Verification items for this drawing (mm, ordinates from the low corner). Round coordinates to 2 decimals unless told otherwise and drop trailing zeros. Order: outer loops, then holes, each group sorted by start corner. A loop starts at its lowest first (then second) coordinate and runs counter-clockwise, first axis right, second up. Notation, with made-up numbers: (-33.5, 84) - (-23.5, 84) arc R31 ccw to (-23.5, 117) - close; hole circle Ø8 at (38, -18.5). An arc over 180 degrees is marked (long way). Use a Markdown table: item, result. Add a question column.
(1) Gauge pin test, flat end, axial feed: P1, Ø10, axis at x = 15, y = 10, coming from the +Z side. Record the tip position at first contact, or that the pin passes through.
(2) Section check B-B on z = 56.5. Record the boundary of the cut face in (x, y).
(3) Section check C-C on y = 40.5. Record the boundary of the cut face in (x, z).
(4) Section check A-A on x = 70.5. Record the boundary of the cut face in (y, z), then the cut area to 3 significant figures.
(5) Mould release check, pull along Z, two halves, no side actions. Record for the marked faces 1, 2, 3 and 4: released by +Z, released by -Z, zero draft, split by the parting line, or undercut.
(6) Section check D-D on x = 82. Record the boundary of the cut face in (y, z) (1 decimal).
(7) Thickness scan on line 1 along Z through (x, y) = (49, 36) (1 decimal); line 2 along X through (y, z) = (35.5, 25); line 3 along X through (y, z) = (27, 61.5) (1 decimal). Record the ranges inside material, lowest first. Write a range as [from, to].
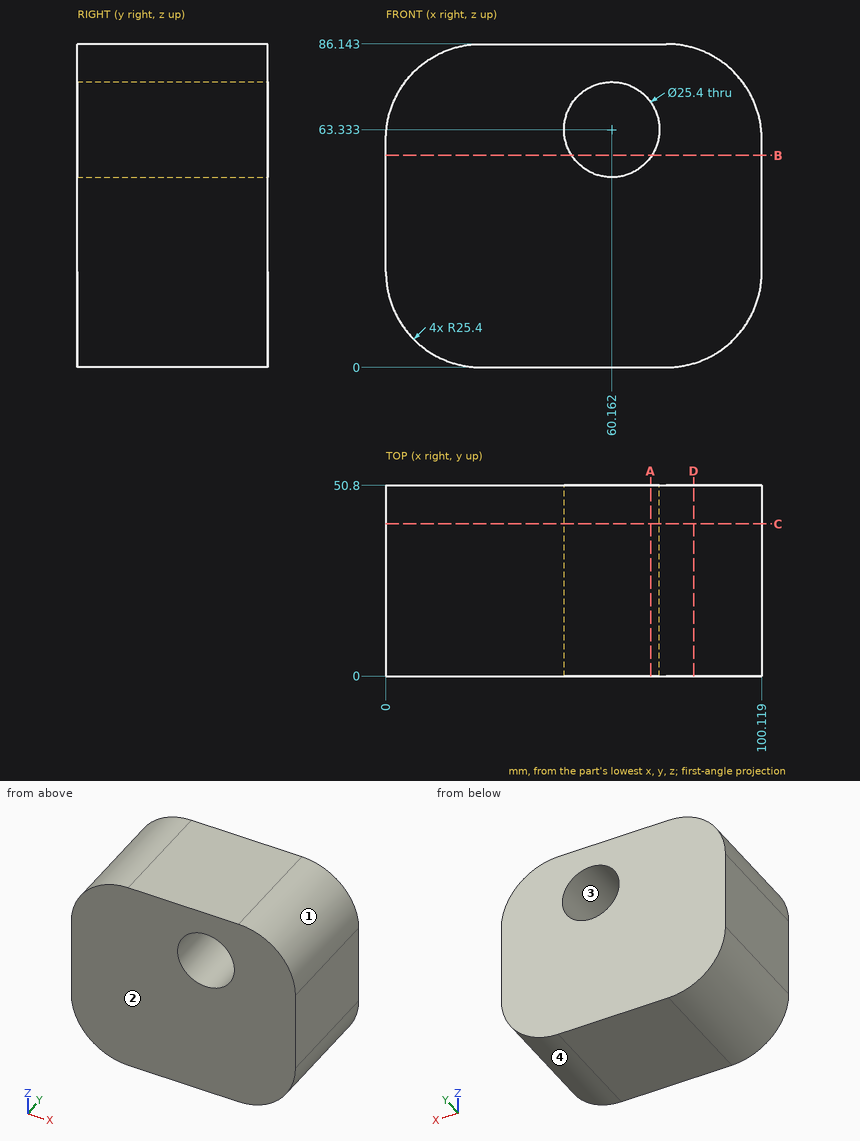
Check sheet entries:
| question | item | result |
|---|---|---|
| 1 | P1 | stops at z = 85.56 |
| 2 | outline | (0, 0) - (49.46, 0) - (49.46, 50.8) - (0, 50.8) - close; (70.87, 0) - (100.12, 0) - (100.12, 50.8) - (70.87, 50.8) - close |
| 3 | outline | (0, 25.4) arc R25.4 ccw to (25.4, 0) - (74.72, 0) arc R25.4 ccw to (100.12, 25.4) - (100.12, 60.74) arc R25.4 ccw to (74.72, 86.14) - (25.4, 86.14) arc R25.4 ccw to (0, 60.74) - close; hole circle Ø25.4 at (60.16, 63.33) |
| 4 | outline | (0, 0) - (50.8, 0) - (50.8, 55.96) - (0, 55.96) - close; (0, 70.71) - (50.8, 70.71) - (50.8, 86.14) - (0, 86.14) - close |
| 4 | area | 3,630 mm2 |
| 5 | face 1 | released by +Z |
| 5 | face 2 | zero draft |
| 5 | face 3 | undercut |
| 5 | face 4 | released by -Z |
| 6 | outline | (0, 1.1) - (50.8, 1.1) - (50.8, 85.1) - (0, 85.1) - close |
| 7 | line 1 | z = [0, 57.3], [69.4, 86.1] |
| 7 | line 2 | x = [0, 100.12] |
| 7 | line 3 | x = [0, 47.6], [72.7, 100.1] |
